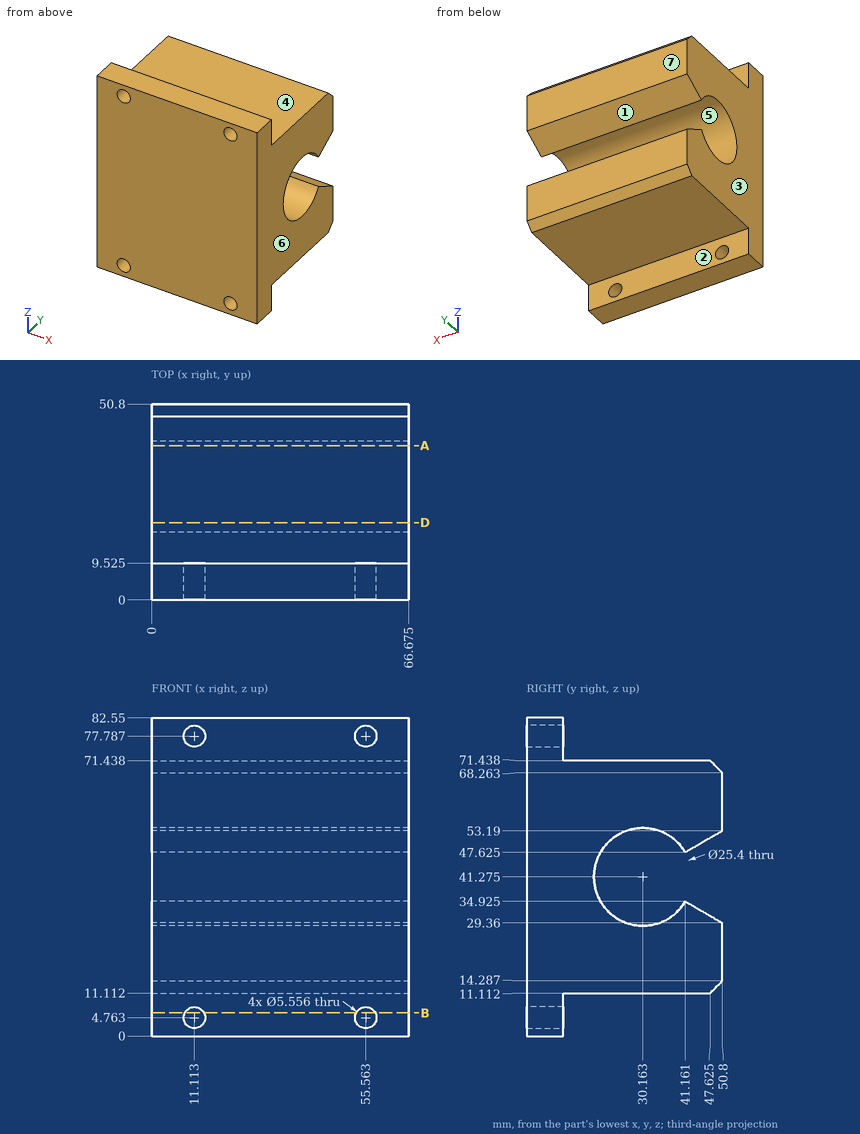
Could you check a few things on this drawing? It's one solid part, dimensions in mm from its lowest x, y, z. A direction names the side the tool comes from. Coordinates: 2 decimals unless noted, no trailing zeros. Order: outer loops, then holes, each group sorted by start corner. A loop starts at its lowest first (then second) coordinate and runs counter-clockwise, first axis right, second up. Notation, with made-up numbers: M 67,-36 L 72,-36 A4 cw 72,-32 Z; hole C 51,-11.5 d11. An arc over 180 degrees is marked long. Use a Markdown table: item, result. Add a question column.
Q1. I want a section at A-A on y = 40. List the corners of the cut face in (x, z) for me (1 decimal), then the cut area to 3 significant figures.
Q2. I'm going to push flat-ended pins straight in: pin 1 (9 mm diameter, centred on x = 11.11, z = 77.79, fed in from +Y) (1 decimal); pin 2 (19 mm diameter, centred on x = 20.5, y = 23.5, fed in from +Z); pin 3 (12 mm diameter, centred on x = 22, z = 76, fed in from +Y); pin 4 (1.5 mm diameter, centred on y = 23, z = 49.5, fed in from -X). Where does each tip first touch, or does it pass through?
Q3. We'd pull the mould along Y, two halves only. Please class the marked faces 5, 6 and 7: pulls with the +Y half, pulls with the -Y half, needs draft (parallel to the pull), parting line crosses it, or undercut.
Q4. If I drill on L1, parallel to Z at x = 60.5, y = 30.5; L2, parallel to Y at x = 37, z = 76 (1 decimal); L3, parallel to Z at x = 21, y = 31.5 (1 decimal), over which ranges is the centre line in solid material (lowest first)?
Q5. I want a section at B-B on z = 6. Give the number of separate pieces and of enclosed holes in the cut face, then the cut area to 3 significant figures.
Q6. Which directions (+Z, -Z, +X, -X, +Y, -Y) give clear straight access to the entire face, cutting with the end or side of a thin tool? Please do the marked faces 1, 2, 3 and 4.
Q7. I want a section at D-D on y = 20. List the corners of the cut face in (x, z) for me (1 decimal), then the cut area to 3 significant figures.
Checked values:
| question | item | result |
|---|---|---|
| 1 | outline | M 0,11.1 L 66.7,11.1 L 66.7,33.2 L 0,33.2 Z; M 0,49.3 L 66.7,49.3 L 66.7,71.4 L 0,71.4 Z |
| 1 | area | 2,950 mm² |
| 2 | pin 1 | y = 9.5 |
| 2 | pin 2 | z = 71.44 |
| 2 | pin 3 | y = 49.06 |
| 2 | pin 4 | through |
| 3 | face 5 | undercut |
| 3 | face 6 | needs draft |
| 3 | face 7 | pulls with the +Y half |
| 4 | L1 | 11.11 to 28.58, 53.97 to 71.44 |
| 4 | L2 | 0 to 9.5 |
| 4 | L3 | 11.1 to 28.6, 53.9 to 71.4 |
| 5 | separate pieces | 3 |
| 5 | enclosed holes | 0 |
| 5 | area | 540 mm² |
| 6 | face 1 | +X, -X, +Y |
| 6 | face 2 | -Z, +X, -X, +Y |
| 6 | face 3 | +Z, -Z, -X, +Y, -Y |
| 6 | face 4 | +Z, +X, -X, +Y |
| 7 | outline | M 0,11.1 L 66.7,11.1 L 66.7,33.7 L 0,33.7 Z; M 0,48.9 L 66.7,48.9 L 66.7,71.4 L 0,71.4 Z |
| 7 | area | 3,010 mm² |
